Source: CAD feature listing. Evaluate the final solid. Frame: model axes, mm. Face numbers are marked on the shaded views. A direction names the side the tool comes from. Give positions to 0.01 mm unless a question says otherwise; leave off trailing zeros. Loops run counter-clockwise (first coordinate to the right, second up) from the corner with the lowest first, then second, coordinate; pieces in that order, holes last. Notation, with made-up numbers: (1, 4.25) -> (54, 4.25) arc R28 cw to (54, 36.25) -> close; hole circle Ø6 at (64, 41.25). An arc over 180 degrees is marked (long way). Return JSON: item names as keys, results as strings. Group by question number.
Autodesk Inventor part; units mm, degrees
ref_plane "YZ Plane" through (0, 0, 0) normal (1, 0, 0) x (0, 1, 0)
ref_plane "XZ Plane" through (0, 0, 0) normal (0, 1, 0) x (-1, 0, 0)
ref_plane "XY Plane" through (0, 0, 0) normal (0, 0, 1) x (1, 0, 0)
sketch "スケッチ1" plane through (0, 0, 0) normal (0, 0, 1) x (1, 0, 0)
  circle A0 centre (0, 0) radius 46
  circle A1 centre (0, 0) radius 50
  circle A2 centre (0, 0) radius 42
  line L0 (0, 0) -> (0, 54.8528)
  line L1 (0, 0) -> (-20.7697, 50.1426)
  circle A3 centre (-17.6034, 42.4985) radius 1.6
  circle A4 centre (-42.4985, 17.6034) radius 1.6
  circle A5 centre (-42.4985, -17.6034) radius 1.6
  circle A6 centre (-17.6034, -42.4985) radius 1.6
  circle A7 centre (17.6034, -42.4985) radius 1.6
  circle A8 centre (42.4985, -17.6034) radius 1.6
  circle A9 centre (42.4985, 17.6034) radius 1.6
  circle A10 centre (17.6034, 42.4985) radius 1.6
  line L2 (0, 0) -> (-55.1659, -46.2897)
  line L3 (-55.1659, -46.2897) -> (-55.1659, 46.2897)
  line L4 (-55.1659, 46.2897) -> (0, 0)
  line L5 (0, 0) -> (-76.7662, 0)
  circle A11 centre (-42.4985, 17.6034) radius 5
  circle A12 centre (-42.4985, -17.6034) radius 5
  point P0 (-32.1739, -26.9971)
  point P1 (-32.1739, 26.9971)
  point P2 (-38.3022, 32.1394)
  point P3 (-38.3022, -32.1394)
  point P4 (-44.9073, -21.985)
  point P5 (-47.2999, -16.2085)
  point P6 (-39.8089, -13.3884)
  point P7 (-37.6162, -18.6821)
  point P8 (-39.8089, 13.3884)
  point P9 (-37.6162, 18.6821)
  point P10 (-47.2999, 16.2085)
  point P11 (-44.9073, 21.985)
  dimension "d0" = 92
  dimension "d1" = 100
  dimension "d2" = 84
  dimension "d3" = 22.5
  dimension "d4" = 3.2
  dimension "d7" = 360
  dimension "d9" = 80
  dimension "d10" = 40
  dimension "d18" = 10
  dimension "d19" = 10
extrude "押し出し1" add sketch "スケッチ1" along normal blind 10 contours L2 A1 A12 A0 | A0 A12 A2 L2 | A2 A11 A0 L4 | L5 A0 A11 A2 | A2 A12 A0 L5 | L4 A0 A11 A1 | A12 A1 A0 A5 | A0 A5 A12 A2 | A2 A12 | A11 A2 | A2 A11 A0 A4 | L5 A1 A11 A0 | A0 A12 A1 L5 | A12 A1 | A11 A0 A4 A1 | A1 A11
fillet "フィレット1" radius 4 4 edges at (-32.1739, -26.9971, 5) (-38.3022, -32.1394, 5) (-38.3022, 32.1394, 5) (-32.1739, 26.9971, 5)
sketch "スケッチ2" plane through (0, 0, 10) normal (0, 0, 1) x (1, 0, 0)
  circle A0 centre (-42.4985, -17.6034) radius 1.6
  circle A1 centre (-42.4985, -17.6034) radius 3
  circle A2 centre (-42.4985, 17.6034) radius 1.6
  circle A3 centre (-42.4985, 17.6034) radius 3
  point P0 (0, 0)
  dimension "d14" = 6
  dimension "d15" = 6
extrude "押し出し2" cut sketch "スケッチ2" against normal blind 5 contours A0 | A1 | A2 | A3
equation "\"d10\" = 0.5 * d9"
properties part number "RP_Hip-Link-Limit-short" material "ABS プラスチック"
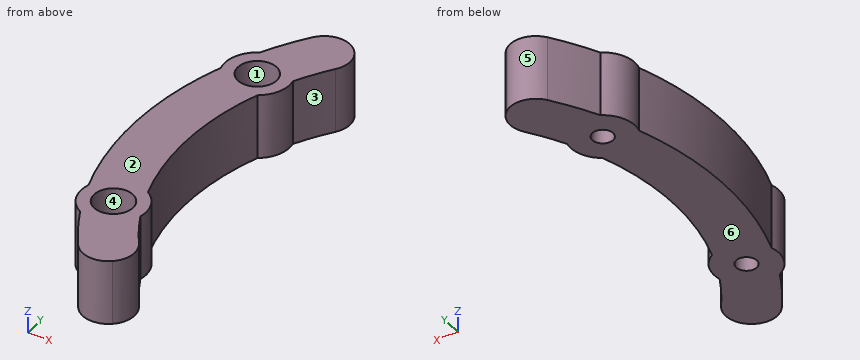
1) Material intervals for line 1 (Z direction, x = -41.75, y = 16); line 2 (X direction, y = -19, z = 8.5); line 3 (X direction, y = 16, z = 8), sorted ascending.
2) Contact query for flat-ended pins moving along their axis: P1, Ø3, axis at y = 0, z = 3.5, coming from the +X side; P2, Ø4, axis at y = -7, z = 1.5, coming from the -X side; P3, Ø5, axis at x = -43.5, z = 7, coming from the -Y side; P4, Ø6, axis at x = -36.5, y = 4, coming from the -Z side. Output: stop coordinate, or through.
3) Cut plane A-A on z = 2.75. Count the separate pieces of the cut face and the enclosed holes in it, then the cut area to 3 significant figures.
4) Reachability of the marked faces 1, 2 and 3 from +Z, -Z, +X, -X, +Y, -Y: full face, straight path, thin tool, end or side. Return the list, or none.
5) Mould query, pull axis Y, two halves, no side actions, for the marked faces 4, 5 and 6. Classes: released by +Y, released by -Y, zero draft, split by the parting line, or undercut.
6) Cut plane D-D on y = 11. Return loops of the section in (x, z) (3 decimals).
7) Cut plane B-B on y = -10.5. Return loops of the section in (x, z).
Calculated:
{
 "1": {"line 1": "0 to 5", "line 2": "-47.3 to -45.15, -39.84 to -37.46", "line 3": "-47.37 to -45.03, -39.96 to -37.76"},
 "2": {"P1": "x = -41.97", "P2": "x = -49.75", "P3": "y = -28.62", "P4": "through"},
 "3": {"separate pieces": "1", "enclosed holes": "2", "area": "500 mm2"},
 "4": {"face 1": "+Z", "face 2": "+Z, +X, -X, +Y, -Y", "face 3": "+Z, -Z, +X"},
 "5": {"face 4": "undercut", "face 5": "released by +Y", "face 6": "zero draft"},
 "6": {"outline": "(-48.775, 0) -> (-40.534, 0) -> (-40.534, 10) -> (-48.775, 10) -> close"},
 "7": {"outline": "(-48.89, 0) -> (-40.67, 0) -> (-40.67, 10) -> (-48.89, 10) -> close"}
}
